Autodesk Inventor part; units mm, degrees
ref_plane "XZ Plane" through (0, 0, 0) normal (0, 1, 0) x (-1, 0, 0)
ref_plane "XY Plane" through (0, 0, 0) normal (0, 0, 1) x (1, 0, 0)
sketch "Sketch1" plane through (0, 0, 0) normal (0, 1, 0) x (-1, 0, 0)
  line L0 (0, 0) -> (0, -500) construction
  line L1 (-5, 0) -> (-5, -500)
  line L2 (5, -500) -> (5, 0)
  arc A0 (5, 0) -> (-5, 0) centre (0, 0) ccw
  arc A1 (-5, -500) -> (5, -500) centre (0, -500) ccw
  circle A2 centre (0, 0) radius 2
  circle A3 centre (0, -500) radius 2
  point P0 (0, -250)
  dimension "d0" = 500
  dimension "d1" = 10
  dimension "d2" = 4
  dimension "d3" = 4
extrude "Extrusion1" add sketch "Sketch1" along normal blind 4
properties part number "Test_arm_3"
Design review of the part built by this model. Coordinates are the model's own, in mm. Coordinates: 2 decimals unless noted, no trailing zeros. Write each loop counter-clockwise with the first axis right and the second up, starting at its lowest first coordinate (ties: lowest second). Pieces come first, ordered by that corner, then holes. Notation, with made-up numbers: (16, 42.5) - (58, 42.5) arc R20 ccw to (58, 54.5) - close; hole circle Ø2 at (76, 3). An arc over 180 degrees is marked (long way). One line per item, written item: value.
1) Add section A-A (x = 0). State the section outline as (y, z) points.
Answer sheet:
outline: (0, -505) - (4, -505) - (4, -502) - (0, -502) - close; (0, -498) - (4, -498) - (4, -2) - (0, -2) - close; (0, 2) - (4, 2) - (4, 5) - (0, 5) - close
2) Insertion check: pin 1 (5 mm diameter, centred on x = 0, z = -500, fed in from -Y); pin 2 (1.5 mm diameter, centred on x = 1, y = 0.5, fed in from +Z); pin 3 (2.5 mm diameter, centred on x = 0, z = 0, fed in from +Y). Each pin has a flat end and moves straight along its axis. Give the tip position at first contact, or say it passes through.
Answer sheet:
pin 1: stops at y = 0
pin 2: stops at z = 4.99
pin 3: passes through
3) To check wall thickness, follow probe 1 along Z at (x, y) = (0, 2.35); probe 2 along X at (y, z) = (1.3, -500); probe 3 along Z at (x, y) = (1.25, 2.55). State the ranges of each line that lie inside material, in increasing order.
Answer sheet:
probe 1: z = -505 to -502, -498 to -2, 2 to 5
probe 2: x = -5 to -2, 2 to 5
probe 3: z = -504.84 to -501.56, -498.44 to -1.56, 1.56 to 4.84
